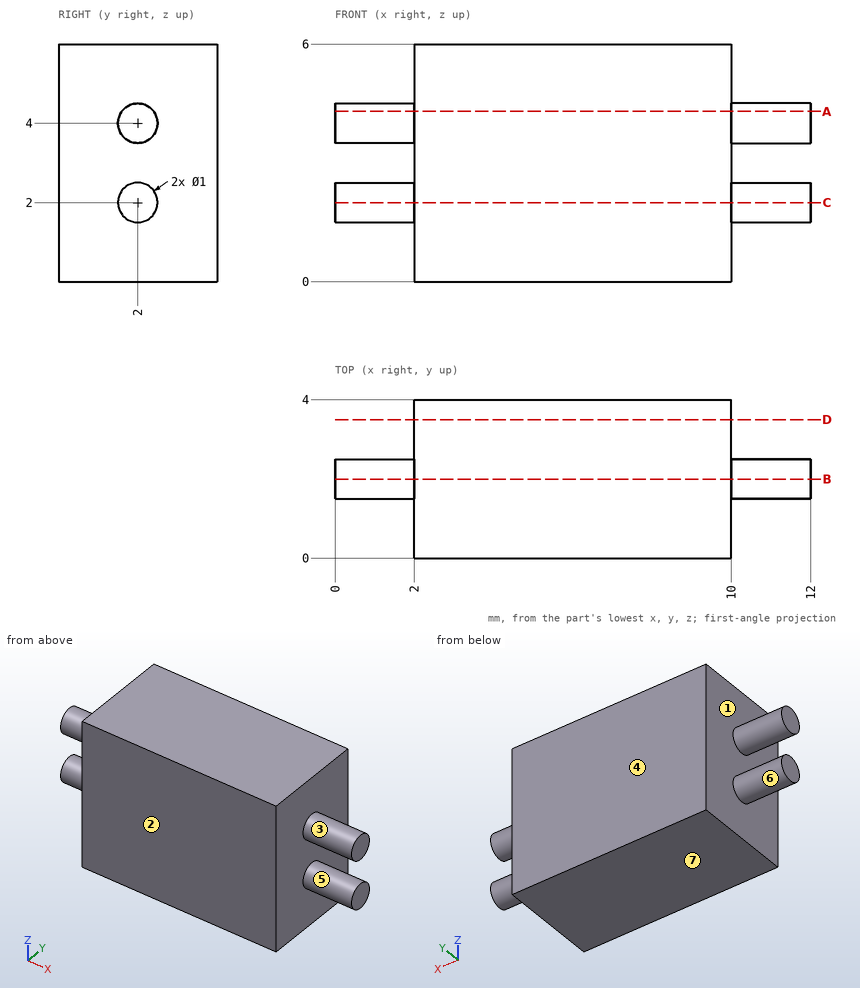
Answer from the drawing. Dimensions are ordinates in mm from the lowest x, y and z of the part. A direction names the side the tool comes from. Coordinates: 2 decimals unless noted, no trailing zeros. Order: outer loops, then holes, each group sorted by start corner. A loop starts at its lowest first (then second) coordinate and runs counter-clockwise, first axis right, second up. Notation, with made-up numbers: (86.5, 2.5) - (145.5, 2.5) arc R21 cw to (145.5, 38.5) - close; hole circle Ø8 at (88, 45.5). An arc over 180 degrees is marked (long way). Put each result on its own line as item: value. Start each with the question number.
1) For a pull along Z with two mould halves and no side action, classify the marked faces 4, 5, 6 and 7 as released by +Z, released by -Z, zero draft, split by the parting line, or undercut.
2) Find section D-D (y = 3.5). Give the vertices of the cut face in (x, z).
3) Find the intervals of material crossed by line 1 (X direction, y = 3.8, z = 1.05), in increasing order. Write a range as from..to.
4) Find section C-C (z = 2). Give the vertices of the cut face in (x, y), plus the area to 3 significant figures.
5) A flat-ended cylindrical pin translates along its axis: pin 1 (1 mm diameter, centred on y = 3.5, z = 0.5, fed in from -X). Find the tip coordinate at first contact, or state that the pin passes through.
6) Find section A-A (z = 4.3). Give the vertices of the cut face in (x, y), plus the area to 3 significant figures.
7) Find section B-B (y = 2). Give the vertices of the cut face in (x, z), plus the area to 3 significant figures.
8) For the marked faces 1, 2 and 3, determine the directions among +Z, -Z, +X, -X, +Y, -Y from which every point of the face is accessible in a straight line to the end or side of a thin tool.
Results list:
1. face 4: zero draft
1. face 5: undercut
1. face 6: undercut
1. face 7: released by -Z
2. outline: (2, 0) - (10, 0) - (10, 6) - (2, 6) - close
3. line 1: x = 2..10
4. outline: (0, 1.5) - (2, 1.5) - (2, 0) - (10, 0) - (10, 1.5) - (12, 1.5) - (12, 2.5) - (10, 2.5) - (10, 4) - (2, 4) - (2, 2.5) - (0, 2.5) - close
4. area: 36.0 mm^2
5. pin 1: stops at x = 2
6. outline: (0, 1.6) - (2, 1.6) - (2, 0) - (10, 0) - (10, 1.6) - (12, 1.6) - (12, 2.4) - (10, 2.4) - (10, 4) - (2, 4) - (2, 2.4) - (0, 2.4) - close
6. area: 35.2 mm^2
7. outline: (0, 1.5) - (2, 1.5) - (2, 0) - (10, 0) - (10, 1.5) - (12, 1.5) - (12, 2.5) - (10, 2.5) - (10, 3.5) - (12, 3.5) - (12, 4.5) - (10, 4.5) - (10, 6) - (2, 6) - (2, 4.5) - (0, 4.5) - (0, 3.5) - (2, 3.5) - (2, 2.5) - (0, 2.5) - close
7. area: 56.0 mm^2
8. face 1: -X
8. face 2: +Z, -Z, +X, -X, -Y
8. face 3: +X
